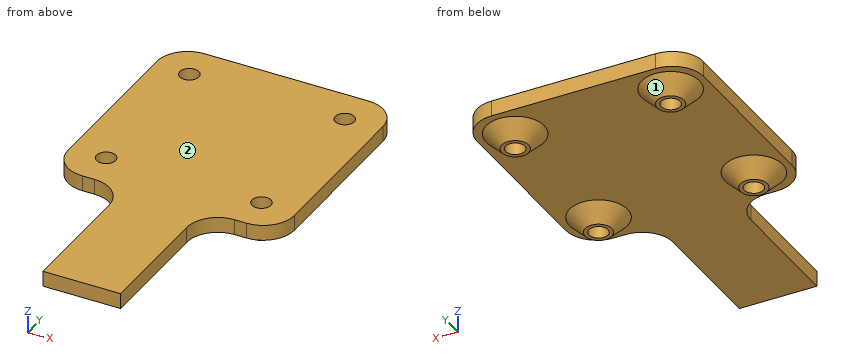
from build123d import *

# Parameters (mm, degrees)
BOSS_EXTRUDE1_DEPTH = 1
SKETCH4_R           = 1.725
SKETCH4_R_2         = 1.225
BOSS_EXTRUDE2_DEPTH = 2
CHAMFER1_SIZE       = 2
FILLET1_R           = 4
CUT_EXTRUDE1_REACH  = 53.265
SKETCH4_2_R         = 1.225


with BuildPart() as part:
    # Sketch3 → Boss-Extrude1 (new, symmetric)
    with BuildSketch(Plane.XY):
        Polygon((5, 19.853558876), (14.56, 19.853558876), (14.56, 49.113558876), (-14.56, 49.113558876), (-14.56, 19.853558876), (-5, 19.853558876), (-5, 0), (5, 0), align=None)
    extrude(amount=BOSS_EXTRUDE1_DEPTH, both=True)

    # Sketch4 → Boss-Extrude2 (add)
    # profile 1 of 4: a face of its own
    with BuildSketch(Plane(origin=(0, 0, -1), x_dir=(-1, 0, 0), z_dir=(0, 0, -1))):
        with Locations((-10, 44.483558876)):
            Circle(SKETCH4_R)
        with Locations((-10, 44.483558876)):
            Circle(SKETCH4_R_2, mode=Mode.SUBTRACT)
    # profile 2 of 4: a face of its own
    with BuildSketch(Plane(origin=(0, 0, -1), x_dir=(-1, 0, 0), z_dir=(0, 0, -1))):
        with Locations((10, 44.483558876)):
            Circle(SKETCH4_R)
        with Locations((10, 44.483558876)):
            Circle(SKETCH4_R_2, mode=Mode.SUBTRACT)
    # profile 3 of 4: a face of its own
    with BuildSketch(Plane(origin=(0, 0, -1), x_dir=(-1, 0, 0), z_dir=(0, 0, -1))):
        with Locations((-10, 24.483558876)):
            Circle(SKETCH4_R)
        with Locations((-10, 24.483558876)):
            Circle(SKETCH4_R_2, mode=Mode.SUBTRACT)
    # profile 4 of 4: a face of its own
    with BuildSketch(Plane(origin=(0, 0, -1), x_dir=(-1, 0, 0), z_dir=(0, 0, -1))):
        with Locations((10, 24.483558876)):
            Circle(SKETCH4_R)
        with Locations((10, 24.483558876)):
            Circle(SKETCH4_R_2, mode=Mode.SUBTRACT)
    extrude(amount=BOSS_EXTRUDE2_DEPTH)

    # Chamfer1
    chamfer1_edges = [part.edges().sort_by_distance(p)[0] for p in [
        (11.725, 44.483558876, -1),
        (-8.275, 44.483558876, -1),
        (11.725, 24.483558876, -1),
        (-8.275, 24.483558876, -1),
    ]]
    chamfer(chamfer1_edges, length=CHAMFER1_SIZE - 0.0001)  # a hair under: the kernel refuses the full size

    # Fillet1
    fillet1_edges = [part.edges().sort_by_distance(p)[0] for p in [
        (-5, 19.853558876, 0),
        (-14.56, 19.853558876, 0),
        (-14.56, 49.113558876, 0),
        (14.56, 49.113558876, 0),
        (14.56, 19.853558876, 0),
        (5, 19.853558876, 0),
    ]]
    fillet(fillet1_edges, radius=FILLET1_R)

    # Sketch4<2> → Cut-Extrude1 (cut, up to next)
    with BuildSketch(Plane(origin=(0, 0, -1), x_dir=(-1, 0, 0), z_dir=(0, 0, -1)), mode=Mode.PRIVATE) as cut_extrude1_sk1:
        with Locations((-10, 44.483558876)):
            Circle(SKETCH4_2_R)
    cut_extrude1_tool1 = extrude(cut_extrude1_sk1.sketch, amount=-CUT_EXTRUDE1_REACH, mode=Mode.PRIVATE) & part.part
    # Sketch4<2> → Cut-Extrude1 (cut, up to next)
    with BuildSketch(Plane(origin=(0, 0, -1), x_dir=(-1, 0, 0), z_dir=(0, 0, -1)), mode=Mode.PRIVATE) as cut_extrude1_sk2:
        with Locations((10, 44.483558876)):
            Circle(SKETCH4_2_R)
    cut_extrude1_tool2 = extrude(cut_extrude1_sk2.sketch, amount=-CUT_EXTRUDE1_REACH, mode=Mode.PRIVATE) & part.part
    # Sketch4<2> → Cut-Extrude1 (cut, up to next)
    with BuildSketch(Plane(origin=(0, 0, -1), x_dir=(-1, 0, 0), z_dir=(0, 0, -1)), mode=Mode.PRIVATE) as cut_extrude1_sk3:
        with Locations((10, 24.483558876)):
            Circle(SKETCH4_2_R)
    cut_extrude1_tool3 = extrude(cut_extrude1_sk3.sketch, amount=-CUT_EXTRUDE1_REACH, mode=Mode.PRIVATE) & part.part
    # Sketch4<2> → Cut-Extrude1 (cut, up to next)
    with BuildSketch(Plane(origin=(0, 0, -1), x_dir=(-1, 0, 0), z_dir=(0, 0, -1)), mode=Mode.PRIVATE) as cut_extrude1_sk4:
        with Locations((-10, 24.483558876)):
            Circle(SKETCH4_2_R)
    cut_extrude1_tool4 = extrude(cut_extrude1_sk4.sketch, amount=-CUT_EXTRUDE1_REACH, mode=Mode.PRIVATE) & part.part
    add(cut_extrude1_tool1.solids().sort_by_distance((10, 44.483559, -1))[0], mode=Mode.SUBTRACT)
    add(cut_extrude1_tool2.solids().sort_by_distance((-10, 44.483559, -1))[0], mode=Mode.SUBTRACT)
    add(cut_extrude1_tool3.solids().sort_by_distance((-10, 24.483559, -1))[0], mode=Mode.SUBTRACT)
    add(cut_extrude1_tool4.solids().sort_by_distance((10, 24.483559, -1))[0], mode=Mode.SUBTRACT)


solid = part.part
Can you work these out from the model? Positions are in its coordinate system, mm. Face numbers are marked on the shaded views. Coordinates: 2 decimals unless noted, no trailing zeros. Loops run counter-clockwise (first coordinate to the right, second up) from the corner with the lowest first, then second, coordinate; pieces in that order, holes last. Notation, with made-up numbers: (-15, 22) - (23, 22) arc R25 cw to (23, 38) - close; hole circle Ø4 at (68, 43). An arc over 180 degrees is marked (long way). Answer as a JSON object with one key per item and string values. Group by question number.
Item 1: If we section it at A-A (x = -10): State how many separate pieces and enclosed holes the cut face has, plus the area to 3 significant figures.
Item 2: If we section it at C-C (y = 8.5): List the corners of the cut face in (x, z) for me, plus the area to 3 significant figures.
Item 3: For pin 1 (1.7 mm diameter, centred on x = -10, z = -0.5, fed in from -Y); pin 2 (1.6 mm diameter, centred on y = 8.5, z = 0, fed in from -X); pin 3 (2 mm diameter, centred on x = 10, y = 44.48, fed in from +Z); pin 4 (0.6 mm diameter, centred on y = 4.5, z = 0, fed in from +X), each with a flat end and sliding along its axis, tell me the tip position at first contact or that it passes through.
Item 4: If we mould it in two halves opening along X, with no side actions, what happens to the marked faces 1 and 2? For each: released by +X, released by -X, zero draft, split by the parting line, or undercut.
Item 5: If we section it at B-B (z = 0.2): List the corners of the cut face in (x, y) for me (3 decimals), plus the area to 3 significant figures.
Item 6: If I drill on L1, parallel to Y at x = -10, z = -0.35; L2, parallel to X at y = 24, z = 0.1; L3, parallel to Y at x = -10.75, z = -1.85 (3 decimals), over which ranges is the centre line in solid material (lowest first)? Write a range as from..to.
Item 7: If we section it at D-D (x = 0.5): List the corners of the cut face in (y, z) for me, plus the area to 3 significant figures.
Returned:
{
 "1": {"separate pieces": "3", "enclosed holes": "0", "area": "60.7 mm²"},
 "2": {"outline": "(-5, -1) - (5, -1) - (5, 1) - (-5, 1) - close", "area": "20.0 mm²"},
 "3": {"pin 1": "stops at y = 19.85", "pin 2": "stops at x = -5", "pin 3": "passes through", "pin 4": "stops at x = 5"},
 "4": {"face 1": "undercut", "face 2": "zero draft"},
 "5": {"outline": "(-14.56, 23.854) arc R4 ccw to (-10.56, 19.854) - (-9, 19.854) arc R4 cw to (-5, 15.854) - (-5, 0) - (5, 0) - (5, 15.854) arc R4 cw to (9, 19.854) - (10.56, 19.854) arc R4 ccw to (14.56, 23.854) - (14.56, 45.114) arc R4 ccw to (10.56, 49.114) - (-10.56, 49.114) arc R4 ccw to (-14.56, 45.114) - close; hole circle Ø2.45 at (-10, 24.484); hole circle Ø2.45 at (-10, 44.484); hole circle Ø2.45 at (10, 24.484); hole circle Ø2.45 at (10, 44.484)", "area": "1,020 mm²"},
 "6": {"L1": "y = 19.85..23.26, 25.71..43.26, 45.71..49.11", "L2": "x = -14.56..-11.13, -8.87..8.87, 11.13..14.56", "L3": "y = 21.708..23.515, 25.452..27.259, 41.708..43.515, 45.452..47.259"},
 "7": {"outline": "(0, -1) - (49.11, -1) - (49.11, 1) - (0, 1) - close", "area": "98.2 mm²"}
}
